from build123d import *

# Parameters (mm, degrees)
F0_W     = 160
F0_H     = 60
F1_DEPTH = 20
F3_DEPTH = 20.001
F4_W     = 80
F4_H     = 60
F5_DEPTH = 40
F6_R     = 8
F7_DEPTH = 120.001
F9_DEPTH = 60.001


with BuildPart() as f1:
    # F0 (on Top) → F1 (new body)
    with BuildSketch(Plane.XY):
        Rectangle(F0_W, F0_H)
    extrude(amount=F1_DEPTH)

    # F2 (on face) → F3 (cut, through all)
    with BuildSketch(Plane.XY.offset(20)):
        with BuildLine():
            ThreePointArc((-71, -15), (-65, -21), (-59, -15))
            Line((-59, -15), (-59, 15))
            ThreePointArc((-59, 15), (-65, 21), (-71, 15))
            Line((-71, 15), (-71, -15))
        make_face()
        with BuildLine():
            ThreePointArc((59, -15), (65, -21), (71, -15))
            Line((71, -15), (71, 15))
            ThreePointArc((71, 15), (65, 21), (59, 15))
            Line((59, 15), (59, -15))
        make_face()
    extrude(amount=-F3_DEPTH, mode=Mode.SUBTRACT)

    # F4 (on face) → F5 (join)
    with BuildSketch(Plane.XY.offset(20)):
        Rectangle(F4_W, F4_H)
    extrude(amount=F5_DEPTH)

    # F6 (on face) → F7 (cut, through all)
    with BuildSketch(Plane.YZ.offset(40)):
        with Locations((0, 45)):
            Circle(F6_R)
    extrude(amount=-F7_DEPTH, mode=Mode.SUBTRACT)

    # F8 (on face) → F9 (cut, through all)
    with BuildSketch(Plane.XZ.offset(30)):
        with BuildLine():
            Line((-30, 60), (30, 60))
            ThreePointArc((30, 60), (0, 90), (-30, 60))
        make_face()
        with BuildLine():
            ThreePointArc((-30, 60), (0, 30), (30, 60))
            Line((30, 60), (-30, 60))
        make_face()
    extrude(amount=-F9_DEPTH, mode=Mode.SUBTRACT)


solid = f1.part
Input: part model. Units: mm. Frame: model coordinates. A direction names the side the tool comes from. Coordinates: 2 decimals unless noted, no trailing zeros. Loops run counter-clockwise (first coordinate to the right, second up) from the corner with the lowest first, then second, coordinate; pieces in that order, holes last.
Q1. Cut plane A-A (x = -65). Output: boundary loops of the cut face in (y, z).
Q2. Set-up query: faces 1 (the face through (32.06, -1.73, 37.19)), 2 (the face through (-56, 0, 20)), 3 (the face through (-65, 21, 10)). Return all of +Z, -Z, +X, -X, +Y, -Y with unobstructed straight access to the full face (end or side cutting, diameter ignored); none if empty.
Q3. Cut plane D-D (z = 34.5). Output: boundary loops of the cut face in (x, y), then the cut area to 3 significant figures.
Q4. Draft query along X for faces 4 (the face through (71, 0, 10)), 5 (the face through (40, 0, 35)), 6 (the face through (35, 0, 60)). Return one class per face: +X half, -X half, draft (parallel to the pull), parting line (faces both ways), or undercut.
Q5. Material intervals for line 1 (X direction, y = 15.5, z = 8.5); line 2 (Z direction, x = -33, y = 0); line 3 (Y direction, x = 34, z = 45), sorted ascending.
Q6. Cut plane B-B (z = 7). Output: boundary loops of the cut face in (x, y).
Q7. Contact query for flat-ended pins moving along their axis: pin 1 (3 mm diameter, centred on x = -56.5, y = -10, fed in from +Z); pin 2 (1.5 mm diameter, centred on y = 9, z = 47, fed in from +X); pin 3 (9.5 mm diameter, centred on y = 0, z = 45, fed in from +X); pin 4 (12 mm diameter, centred on y = -8, z = 32.5, fed in from -X). Output: stop coordinate, or through.
Q8. Cut plane C-C (y = 25). Output: boundary loops of the cut face in (x, z).
Working result:
1. outline: (-30, 0) - (-21, 0) - (-21, 20) - (-30, 20) - close; (21, 0) - (30, 0) - (30, 20) - (21, 20) - close
2. face 1: +X, -X
2. face 2: +Z, -X, +Y, -Y
2. face 3: +Z, -Z
3. outline: (-40, -30) - (-15.8, -30) - (-15.8, 30) - (-40, 30) - close; (15.8, -30) - (40, -30) - (40, 30) - (15.8, 30) - close
3. area: 2,900 mm2
4. face 4: undercut
4. face 5: +X half
4. face 6: draft
5. line 1: x = -80 to -70.98, -59.02 to 59.02, 70.98 to 80
5. line 2: z = 0 to 37, 53 to 60
5. line 3: y = -30 to -8, 8 to 30
6. outline: (-80, -30) - (80, -30) - (80, 30) - (-80, 30) - close; hole (-71, -15) arc R6 ccw to (-59, -15) - (-59, 15) arc R6 ccw to (-71, 15) - close; hole (59, -15) arc R6 ccw to (71, -15) - (71, 15) arc R6 ccw to (59, 15) - close
7. pin 1: stops at z = 20
7. pin 2: stops at x = 40
7. pin 3: passes through
7. pin 4: stops at x = -40
8. outline: (-80, 0) - (80, 0) - (80, 20) - (40, 20) - (40, 60) - (30, 60) arc R30 cw to (-30, 60) - (-40, 60) - (-40, 20) - (-80, 20) - close
